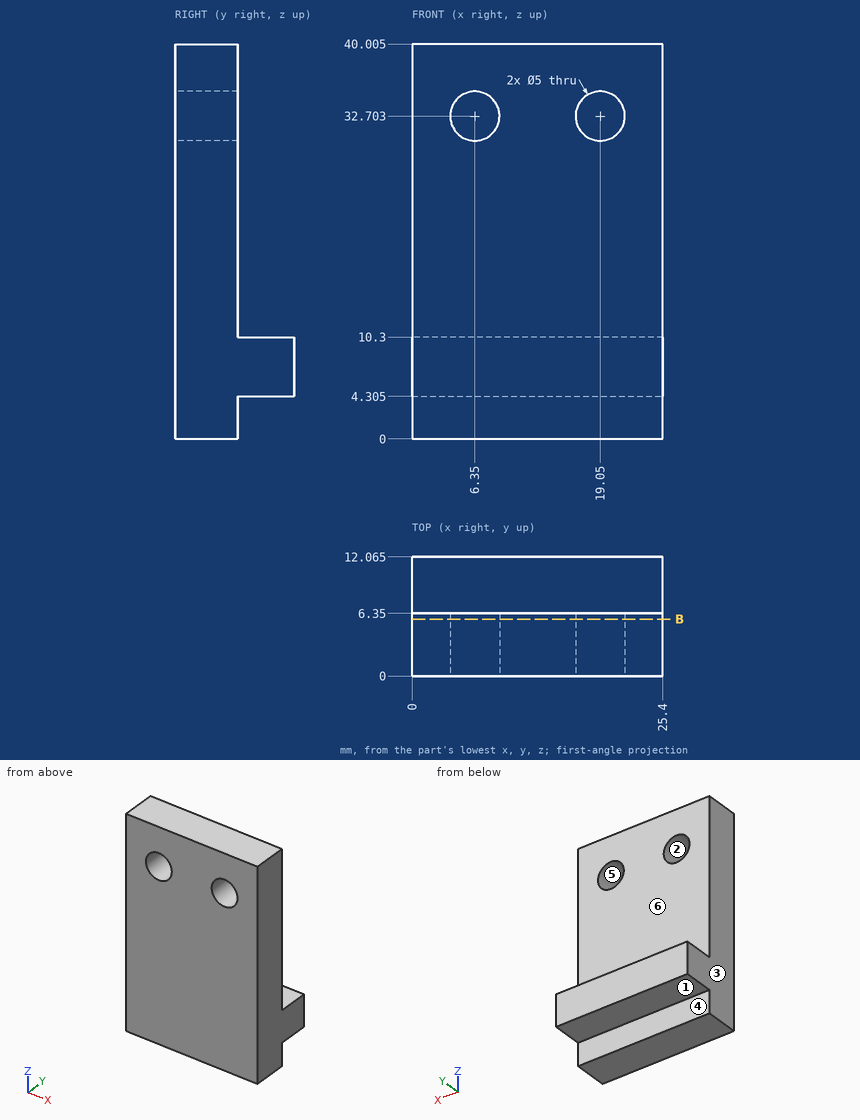
Part print with two shaded views. Sizes in mm from the minimum x, y, z corner. A direction names the side the tool comes from. Coordinates: 2 decimals unless noted, no trailing zeros. One line per item, written item: value. Start each with the question number.
1. Probe line 1 (Z direction, x = 19.05, y = 3.25) (1 decimal); line 2 (Z direction, x = 14.25, y = 9) (1 decimal); line 3 (Y direction, x = 21.25, z = 26). List the from-to ranges inside material, lowest first. Write a range as from..to.
2. Flat gauge pins, fed straight in: pin 1 (6 mm diameter, centred on x = 16, z = 36, fed in from +Y); pin 2 (6.5 mm diameter, centred on x = 8.5, y = 10, fed in from +Z); pin 3 (3 mm diameter, centred on x = 18, y = 8, fed in from -Z) (1 decimal). Where does each tip first touch, or does it go through?
3. Slice it at B-B (y = 5.75). Count the separate pieces of the cut face and the enclosed holes in it, plus the area to 3 significant figures.
4. Mould opens along X. For the marked faces 1, 2 and 3 say: released by +X, released by -X, zero draft, split by the parting line, or undercut.
5. Tool access for the marked faces 4, 5 and 6: list every direction of +Z, -Z, +X, -X, +Y, -Y with a clear straight run to the whole face (end or side of a thin tool).
Answers below:
1. line 1: z = 0..30.2, 35.2..40
1. line 2: z = 4.3..10.3
1. line 3: y = 0..6.35
2. pin 1: stops at y = 6.35
2. pin 2: stops at z = 10.3
2. pin 3: stops at z = 4.3
3. separate pieces: 1
3. enclosed holes: 2
3. area: 977 mm^2
4. face 1: zero draft
4. face 2: undercut
4. face 3: released by -X
5. face 4: -Z, +X, -X, +Y
5. face 5: +Y, -Y
5. face 6: +Z, +X, -X, +Y
